from build123d import *

# Parameters (mm, degrees)
SWEEP1_START       = -30
SWEEP1_OUTLINE_R   = 9
SWEEP1_DEPTH       = 30
SKETCH26_R         = 5
CUT_EXTRUDE1_DEPTH = 15
SKETCH27_R         = 8
CUT_EXTRUDE2_DEPTH = 15


# Read off the part's stored shape, not the designer's step: Sweep1
with BuildPart() as part:
    # Sweep1 outline → Sweep1 (new body)
    with BuildSketch(Plane(origin=(0, 0, 0), x_dir=(1, 0, 0), z_dir=(0, 1, 0)).offset(SWEEP1_START)):
        with Locations((20, 0)):
            Circle(SWEEP1_OUTLINE_R)
    extrude(amount=SWEEP1_DEPTH)

    # Sketch26 → Cut-Extrude1 (cut)
    with BuildSketch(Plane(origin=(0, -30, 0), x_dir=(-1, 0, 0), z_dir=(0, -1, 0))):
        with Locations(Location((-20.053022343, 0, 0), (0, 0, 180))):
            Circle(SKETCH26_R)
    extrude(amount=-CUT_EXTRUDE1_DEPTH, mode=Mode.SUBTRACT)

    # Sketch27 → Cut-Extrude2 (cut)
    with BuildSketch(Plane(origin=(0, 0, 0), x_dir=(1, 0, 0), z_dir=(0, 1, 0))):
        with Locations(Location((20.053022343, 0, 0), (0, 0, 180))):
            Circle(SKETCH27_R)
    extrude(amount=-CUT_EXTRUDE2_DEPTH, mode=Mode.SUBTRACT)


solid = part.part
The model under review builds one solid part; all positions refer to its coordinate system, in mm. A direction names the side the tool comes from. Coordinates: 2 decimals unless noted, no trailing zeros. Write each loop counter-clockwise with the first axis right and the second up, starting at its lowest first coordinate (ties: lowest second). Pieces come first, ordered by that corner, then holes. Notation, with made-up numbers: (50.25, 59) -> (73.25, 59) arc R7 ccw to (73.25, 69) -> close; hole circle Ø11 at (61, 58.5). An arc over 180 degrees is marked (long way). Answer in a Markdown table with one row per item.
1. We need section D-D, the plane x = 12.5. State the section outline as (y, z) points, and give its area (3 significant figures).
Answers below:
| item | result |
|---|---|
| outline | (-30, -4.97) -> (0, -4.97) -> (0, -2.64) -> (-15, -2.64) -> (-15, 2.64) -> (0, 2.64) -> (0, 4.97) -> (-30, 4.97) -> close |
| area | 219 mm^2 |
2. Wall thickness on probe 1 along Y at (x, z) = (12.75, 1.5); probe 2 along X at (y, z) = (-3, 4.5); probe 3 along Z at (x, y) = (17.5, -19.5): over which ranges is each line inside the solid? List them lowest first. Write a range as [from, to].
Answers below:
| item | result |
|---|---|
| probe 1 | y = [-30, -15] |
| probe 2 | x = [12.21, 13.44], [26.67, 27.79] |
| probe 3 | z = [-8.65, -4.3], [4.3, 8.65] |
3. We need section C-C, the plane y = -20.25. State the section outline as (x, z) points.
Answers below:
| item | result |
|---|---|
| outline | circle Ø18 at (20, 0); hole circle Ø10 at (20.05, 0) |
4. We need section A-A, the plane z = 0. State the section outline as (x, y) points.
Answers below:
| item | result |
|---|---|
| outline | (11, -30) -> (15.05, -30) -> (15.05, -15) -> (12.05, -15) -> (12.05, 0) -> (11, 0) -> close; (25.05, -30) -> (29, -30) -> (29, 0) -> (28.05, 0) -> (28.05, -15) -> (25.05, -15) -> close |
5. Clearance check with flat-ended pins moving along their axes: pin 1 Ø6 at (y, z) = (-21, -4) entering from -X; pin 2 Ø1 at (y, z) = (-7.5, 6.5) entering from +X; pin 3 Ø10 at (y, z) = (-4.5, 5.5) entering from +X. State where each tip first meets the part, or that it passes through.
Answers below:
| item | result |
|---|---|
| pin 1 | stops at x = 11.06 |
| pin 2 | stops at x = 26.71 |
| pin 3 | stops at x = 28.99 |
6. Draft analysis for pull direction X (two halves, no side actions). For faces 3 (the cylindrical face through (24.822, -22.605, 1.502)), 4 (the flat face through (24, -30, 4)), 5 (the cylindrical face through (28.584, -15.21, -2.703)), 6 (the flat face through (14.8, -15, 0.1)), state which applies: +X half, -X half, draft (parallel to the pull), parting line (faces both ways), or undercut.
Answers below:
| item | result |
|---|---|
| face 3 | undercut |
| face 4 | draft |
| face 5 | parting line |
| face 6 | undercut |
7. We need section B-B, the plane x = 21.25. State the section outline as (y, z) points.
Answers below:
| item | result |
|---|---|
| outline | (-30, -8.91) -> (0, -8.91) -> (0, -7.91) -> (-15, -7.91) -> (-15, -4.85) -> (-30, -4.85) -> close; (-30, 4.85) -> (-15, 4.85) -> (-15, 7.91) -> (0, 7.91) -> (0, 8.91) -> (-30, 8.91) -> close |
8. For faces 1 (the cylindrical face through (26.4, -7.4, -4.87)), 2 (the flat face through (12.6, 0, 3.3)), list the 3-axis set-ups (+Z, -Z, +X, -X, +Y, -Y) from which the entire face can be reached by the end or side of a thin tool; tool diameter is ignored.
Answers below:
| item | result |
|---|---|
| face 1 | +Y |
| face 2 | +Z, -Z, +X, -X, +Y |
